from build123d import *

# Parameters (mm, degrees)
F1_DEPTH = 3.2766
F3_DEPTH = 7.62
F4_R     = 14.2875
F5_DEPTH = 9.906
F6_R     = 0.772384
F7_DEPTH = 15.5575


with BuildPart() as f1:
    # F0 (on Top) → F1 (new body)
    with BuildSketch(Plane.XY):
        with BuildLine():
            Line((8.256221, 20.6756), (-8.256221, 20.6756))
            ThreePointArc((-8.256221, 20.6756), (-15.742389, 15.742389), (-20.6756, 8.256221))
            Line((-20.6756, 8.256221), (-20.6756, -8.256221))
            ThreePointArc((-20.6756, -8.256221), (-15.742389, -15.742389), (-8.256221, -20.6756))
            Line((-8.256221, -20.6756), (8.256221, -20.6756))
            ThreePointArc((8.256221, -20.6756), (15.742389, -15.742389), (20.6756, -8.256221))
            Line((20.6756, -8.256221), (20.6756, 8.256221))
            ThreePointArc((20.6756, 8.256221), (15.742389, 15.742389), (8.256221, 20.6756))
        make_face()
    extrude(amount=F1_DEPTH)

    # F2 (on face) → F3 (join)
    with BuildSketch(Plane.XY.offset(3.2766)):
        with BuildLine():
            Line((-6.35, -14.549678), (6.35, -14.549678))
            ThreePointArc((6.35, -14.549678), (0, 15.875), (-6.35, -14.549678))
        make_face()
    extrude(amount=F3_DEPTH)

    # F4 (on face) → F5 (join)
    with BuildSketch(Plane.XY.offset(10.8966)):
        Circle(F4_R)
    extrude(amount=F5_DEPTH)

    # F6 (on Front) → F7 (join)
    with BuildSketch(Plane.XZ):
        with Locations((0, 18.963106)):
            Circle(F6_R)
    extrude(amount=-F7_DEPTH)


solid = f1.part
Part model, mm, in its own coordinate system. A direction names the side the tool comes from. Give positions to 0.01 mm unless a question says otherwise; leave off trailing zeros. Loops run counter-clockwise (first coordinate to the right, second up) from the corner with the lowest first, then second, coordinate; pieces in that order, holes last. Notation, with made-up numbers: M -0.75,0.25 L 32.25,0.25 A35 cw 32.25,37.25 Z; hole C 1.5,-17 d5. An arc over 180 degrees is marked long. Put each result on its own line as item: value. Start each with the question number.
1) Saw through at C-C (z = 7.25). List the corners of the cut face in (x, y) (3 decimals).
2) Probe probe 1 along Z at (x, y) = (-15, -9); probe 2 along Z at (x, y) = (-1.5, 14.5); probe 3 along Y at (x, z) = (-12, 12). List the from-to ranges inside material, lowest first.
3) Saw through at A-A (y = 0). List the corners of the cut face in (x, z) (1 decimal), then the cut area to 3 significant figures.
4) Flat gauge pins, fed straight in: pin 1 (3 mm diameter, centred on y = 9, z = 13, fed in from -X); pin 2 (1 mm diameter, centred on x = -3.5, z = 7.5, fed in from -Y); pin 3 (1 mm diameter, centred on y = -7, z = 15, fed in from -X). Where does each tip first touch, or does it go through?
5) Saw through at D-D (y = 12.5). List the corners of the cut face in (x, z), then the cut area to 3 significant figures.
6) 3-axis set-ups, long thin cutter, end or side, ignore diameter. For faces 1 (the cylindrical face through (0.607, 15.863, 7.033)), 2 (the flat face through (0, 15.558, 19)), 3 (the flat face through (0, -20.676, 2)): which of +Z, -Z, +X, -X, +Y, -Y reach the whole face in a straight line?
7) Pull direction Z, two halves, no side cores. Call faces 4 (the cylindrical face through (0.36, 14.9, 18.28)), 5 (the flat face through (0, -14.55, 7)), 6 (the flat face through (0, 0, 0)): +Z half, -Z half, draft (parallel to the pull), parting line (faces both ways), or undercut.
Numbers:
1. outline: M -6.35,-14.55 L 6.35,-14.55 A15.875 ccw long Z
2. probe 1: 0 to 3.28
2. probe 2: 0 to 10.9
2. probe 3: -7.75 to 7.75
3. outline: M -20.7,0 L 20.7,0 L 20.7,3.3 L 15.9,3.3 L 15.9,10.9 L 14.3,10.9 L 14.3,20.8 L -14.3,20.8 L -14.3,10.9 L -15.9,10.9 L -15.9,3.3 L -20.7,3.3 Z
3. area: 660 mm^2
4. pin 1: x = -12.16
4. pin 2: y = -14.55
4. pin 3: x = -12.72
5. outline: M -18.42,0 L 18.42,0 L 18.42,3.28 L 9.79,3.28 L 9.79,10.9 L 6.92,10.9 L 6.92,20.8 L -6.92,20.8 L -6.92,10.9 L -9.79,10.9 L -9.79,3.28 L -18.42,3.28 Z
5. area: 407 mm^2
6. face 1: +Z
6. face 2: +Z, +X, -X, +Y
6. face 3: +Z, -Z, +X, -X, -Y
7. face 4: undercut
7. face 5: draft
7. face 6: -Z half
